```python
from build123d import *

# Parameters (mm, degrees)
F0_R     = 27
F0_R_2   = 25
F1_DEPTH = 20
F2_R     = 27
F3_DEPTH = 2
F4_W     = 35
F4_H     = 4
F5_DEPTH = 25


with BuildPart() as f1:
    # F0 (on Top) → F1 (new body)
    with BuildSketch(Plane.XY):
        Circle(F0_R)
        Circle(F0_R_2, mode=Mode.SUBTRACT)
    extrude(amount=F1_DEPTH)

    # F2 (on face) → F3 (join)
    with BuildSketch(Plane.XY.offset(20)):
        Circle(F2_R)
    extrude(amount=F3_DEPTH)

    # F4 (on face) → F5 (join)
    with BuildSketch(Plane.XY.offset(22)):
        Rectangle(F4_W, F4_H)
    extrude(amount=F5_DEPTH)


solid = f1.part
```
Model file for the job. Use its own axes, mm. A direction names the side the tool comes from. Coordinates: 2 decimals unless noted, no trailing zeros. Loops run counter-clockwise (first coordinate to the right, second up) from the corner with the lowest first, then second, coordinate; pieces in that order, holes last. Notation, with made-up numbers: (-17, 57) - (18, 57) arc R19 cw to (18, 92) - close; hole circle Ø3 at (1.5, 62). An arc over 180 degrees is marked (long way). Answer as a JSON object with one key per item and string values. Group by question number.
(1) Probe line 1 along Y through (x, z) = (0, 10.5); line 2 along Z through (x, y) = (-12, -10); line 3 along Y through (x, z) = (-17, 35.5). List the from-to ranges inside material, lowest first.
(2) Tool access for faces 1 (the face through (0, 2, 34)), 2 (the face through (-5.85, -26.36, 10.85)), 3 (the face through (17.5, 0, 34)), 4 (the face through (-17.5, 0, 34)): list every direction of +Z, -Z, +X, -X, +Y, -Y with a clear straight run to the whole face (end or side of a thin tool).
(3) Two-plate mould, pull along Y, no slides. Class faces 5 (the face through (0, 0, 20)), 6 (the face through (0, -2, 34)), 7 (the face through (24, -8, 0)), 8 (the face through (23.846, 7.509, 9.86)): released by +Y, released by -Y, zero draft, split by the parting line, or undercut.
(4) Cut at A-A (y = 0). Give the cut face in (x, z), then the cut area to 3 significant figures.
(5) Cut at B-B (x = 0). Give the cut face in (y, z).
(6) Cut at D-D (x = 19.5). Give the cut face in (y, z).
(7) Cut at C-C (z = 29). Give the cut face in (x, y), then the cut area to 3 significant figures.
(8) Flat gauge pins, fed straight in: pin 1 (3 mm diameter, centred on x = -9, z = 17, fed in from +Y); pin 2 (2 mm diameter, centred on y = -0.5, z = 40, fed in from +X); pin 3 (3 mm diameter, centred on y = -3.5, z = 20.5, fed in from +X). Where does each tip first touch, or does it go through?
Geometry says:
{
 "1": {"line 1": "y = -27 to -25, 25 to 27", "line 2": "z = 20 to 22", "line 3": "y = -2 to 2"},
 "2": {"face 1": "+Z, +X, -X, +Y", "face 2": "+Z, -Z", "face 3": "+Z, +X, +Y, -Y", "face 4": "+Z, -X, +Y, -Y"},
 "3": {"face 5": "undercut", "face 6": "released by -Y", "face 7": "zero draft", "face 8": "undercut"},
 "4": {"outline": "(-27, 0) - (-25, 0) - (-25, 20) - (25, 20) - (25, 0) - (27, 0) - (27, 22) - (17.5, 22) - (17.5, 47) - (-17.5, 47) - (-17.5, 22) - (-27, 22) - close", "area": "1,060 mm^2"},
 "5": {"outline": "(-27, 0) - (-25, 0) - (-25, 20) - (25, 20) - (25, 0) - (27, 0) - (27, 22) - (2, 22) - (2, 47) - (-2, 47) - (-2, 22) - (-27, 22) - close"},
 "6": {"outline": "(-18.67, 0) - (-15.64, 0) - (-15.64, 20) - (15.64, 20) - (15.64, 0) - (18.67, 0) - (18.67, 22) - (-18.67, 22) - close"},
 "7": {"outline": "(-17.5, -2) - (17.5, -2) - (17.5, 2) - (-17.5, 2) - close", "area": "140 mm^2"},
 "8": {"pin 1": "stops at y = 25.94", "pin 2": "stops at x = 17.5", "pin 3": "stops at x = 26.93"}
}
